Model file for the job. Use its own axes, mm. A direction names the side the tool comes from. Round coordinates to 2 decimals unless told otherwise and drop trailing zeros. Order: outer loops, then holes, each group sorted by start corner. A loop starts at its lowest first (then second) coordinate and runs counter-clockwise, first axis right, second up. Notation, with made-up numbers: M 19,46.25 L 65,46.25 A20 ccw 65,80.25 Z; hole C -34,0.25 d2. An arc over 180 degrees is marked long. Return JSON: item names as keys, results as strings. Group by question number.
Item 1: Slice it at A-A on x = 0.5. Write the cut outline in (y, z).
Item 2: Pin check, flat tips, straight feed: pin 1 Ø10 at (x, z) = (3.5, 30) entering from +Y; pin 2 Ø16 at (y, z) = (10, 29.5) entering from +X; pin 3 Ø9 at (x, z) = (0, 25.5) entering from +Y. Stop position of each tip, or through.
Item 3: Slice it at B-B on y = 11.5. Write the cut outline in (x, z), then the cut area to 3 significant figures.
Item 4: Slice it at D-D on x = 11. Write the cut outline in (y, z), then the cut area to 3 significant figures.
Item 5: Which spindle directions (+Z, -Z, +X, -X, +Y, -Y) get a long thin tool onto all of the face, cutting with end or side? Do faces 1 (the face through (15, -5, 30)), 2 (the face through (13, 10, 10)), 3 (the face through (0, 0, 0)). Say none if no direction does.
Item 6: Pull direction X, two halves, no side cores. Call faces 4 (the face through (-7, 10, 18)), 5 (the face through (-10, 15, 15)), 6 (the face through (-5, -5, 30)): pulls with the +X half, pulls with the -X half, needs draft (parallel to the pull), parting line crosses it, or undercut.
Item 7: Probe line 1 along Y through (x, z) = (19, 37.5); line 2 along Y through (x, z) = (17, 25.5); line 3 along X through (y, z) = (6.5, 32.5). List the from-to ranges inside material, lowest first.
Item 8: Slice it at C-C on z = 22.5. Write the cut outline in (x, y), then the cut area to 4 significant figures.
Autodesk Inventor part; units mm, degrees
ref_plane "YZ Plane" through (0, 0, 0) normal (1, 0, 0) x (0, 1, 0)
ref_plane "XZ Plane" through (0, 0, 0) normal (0, 1, 0) x (-1, 0, 0)
ref_plane "XY Plane" through (0, 0, 0) normal (0, 0, 1) x (1, 0, 0)
sketch "草圖1" plane through (0, 0, 0) normal (0, 0, 1) x (1, 0, 0)
  line L0 (25, -20) -> (-25, -20)
  line L1 (-25, -20) -> (-25, 20)
  line L2 (-25, 20) -> (25, 20)
  line L3 (25, 20) -> (25, -20)
  line L4 (25, -20) -> (-25, 20) construction
  line L5 (-25, -20) -> (25, 20) construction
  point P0 (0, 0)
  dimension "d0" = 40
  dimension "d1" = 50
extrude "擠出1" add sketch "草圖1" along normal blind 40
sketch "草圖2" plane through (-25, 20, 0) normal (0, 1, 0) x (1, 0, 0)
  line L0 (50, -40) -> (0, -40)
  line L1 (50, 0) -> (50, -40)
  line L2 (0, 0) -> (0, -40)
  line L3 (50, 0) -> (0, 0)
  line L4 (0, -40) -> (50, -40)
  line L5 (50, -40) -> (30, -20)
  line L6 (30, -20) -> (10, -40)
  line L7 (10, -40) -> (50, -40)
  line L8 (50, 0) -> (0, 0)
  line L9 (0, 0) -> (0, -40)
  line L10 (50, -40) -> (0, -40)
  line L11 (50, 0) -> (50, -40)
  point P0 (25, 0)
  dimension "d4" = 10
  dimension "d5" = 20
  dimension "d6" = 20
extrude "擠出2" cut sketch "草圖2" against normal blind 30 contours L0 L6 L5
sketch "草圖3" plane through (-25, 20, 0) normal (0, 1, 0) x (1, 0, 0)
  line L0 (0, -40) -> (50, -40)
  line L1 (10, -40) -> (10, -30)
  line L2 (10, -30) -> (30, -10)
  line L3 (30, -10) -> (50, -10)
  line L4 (50, 0) -> (50, -40)
  line L5 (50, 0) -> (0, 0)
  line L6 (0, 0) -> (0, -40)
  point P0 (25, 0)
  dimension "d9" = 10
  dimension "d10" = 10
  dimension "d11" = 10
  dimension "d12" = 20
extrude "擠出3" cut sketch "草圖3" against normal blind 20 contours L1 L2 L3 L4 L0
sketch "草圖4" plane through (-25, 20, 0) normal (0, 1, 0) x (1, 0, 0)
  line L0 (10, -40) -> (10, -30)
  line L1 (10, -30) -> (10, -20)
  line L2 (10, -20) -> (20, -10)
  line L3 (30, -10) -> (50, -10)
  line L4 (20, -10) -> (30, -10)
  line L5 (30, -10) -> (50, -10)
  line L6 (10, -30) -> (30, -10)
  line L7 (10, -30) -> (30, -10)
  point P0 (25, 0)
  dimension "d15" = 10
  dimension "d16" = 10
extrude "擠出4" cut sketch "草圖4" against normal blind 10
Output values:
{
 "1": {"outline": "M -20,0 L 20,0 L 20,10 L 10,10 L 10,14.5 L 0,14.5 L 0,24.5 L -10,24.5 L -10,40 L -20,40 Z"},
 "2": {"pin 1": "y = -10", "pin 2": "x = -6.5", "pin 3": "y = 0"},
 "3": {"outline": "M -25,0 L 25,0 L 25,10 L -5,10 L -15,20 L -15,40 L -25,40 Z", "area": "850 mm²"},
 "4": {"outline": "M -20,0 L 20,0 L 20,10 L 0,10 L 0,26 L -10,26 L -10,40 L -20,40 Z", "area": "860 mm²"},
 "5": {"face 1": "+Z, +Y", "face 2": "+Z, +X, +Y", "face 3": "-Z, +X, -X, +Y, -Y"},
 "6": {"face 4": "needs draft", "face 5": "pulls with the +X half", "face 6": "undercut"},
 "7": {"line 1": "-20 to -10", "line 2": "-20 to 0", "line 3": "-25 to -15"},
 "8": {"outline": "M -25,-20 L 25,-20 L 25,0 L 7.5,0 L 7.5,-10 L 2.5,-10 L 2.5,0 L -7.5,0 L -7.5,10 L -15,10 L -15,20 L -25,20 Z", "area": "1,225 mm²"}
}
